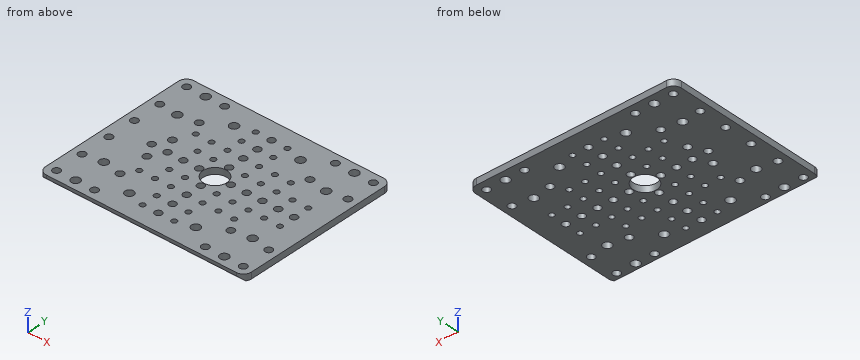
```python
from build123d import *

# Parameters (mm, degrees)
SKETCH_W        = 130
SKETCH_H        = 104
PAD_DEPTH       = 4
SKETCH001_R     = 2.35
SKETCH001_R_2   = 2.75
POCKET_DEPTH    = 4.001
SKETCH002_R     = 1.7
SKETCH002_R_2   = 2.25
SKETCH002_R_3   = 7.5
POCKET001_DEPTH = 5
CHAMFER_SIZE    = 2
FILLET_R        = 5


with BuildPart() as part:
    # Sketch → Pad (new body)
    with BuildSketch(Plane.XY):
        Rectangle(SKETCH_W, SKETCH_H)
    extrude(amount=PAD_DEPTH)

    # Sketch001 → Pocket (cut, through all)
    with BuildSketch(Plane.XY.offset(4)):
        with Locations((-35, 46)):
            Circle(SKETCH001_R)
        with Locations((-59, 27)):
            Circle(SKETCH001_R)
        with Locations((-59, 46)):
            Circle(SKETCH001_R)
        with Locations((35, 46)):
            Circle(SKETCH001_R)
        with Locations((59, 28)):
            Circle(SKETCH001_R)
        with Locations((59, 46)):
            Circle(SKETCH001_R)
        with Locations((59, -28)):
            Circle(SKETCH001_R)
        with Locations((59, -46)):
            Circle(SKETCH001_R)
        with Locations((35, -46)):
            Circle(SKETCH001_R)
        with Locations((-59, -28)):
            Circle(SKETCH001_R)
        with Locations((-35, -46)):
            Circle(SKETCH001_R)
        with Locations((-59, -46)):
            Circle(SKETCH001_R)
        with Locations((-47, 46)):
            Circle(SKETCH001_R_2)
        with Locations((-47, 26)):
            Circle(SKETCH001_R_2)
        with Locations((47, 46)):
            Circle(SKETCH001_R_2)
        with Locations((47, 26)):
            Circle(SKETCH001_R_2)
        with Locations((-21, -37)):
            Circle(SKETCH001_R_2)
        with Locations((21, -37)):
            Circle(SKETCH001_R_2)
        with Locations((-21, 37)):
            Circle(SKETCH001_R_2)
        with Locations((21, 37)):
            Circle(SKETCH001_R_2)
        with Locations((47, -46)):
            Circle(SKETCH001_R_2)
        with Locations((47, -26)):
            Circle(SKETCH001_R_2)
        with Locations((-47, -26)):
            Circle(SKETCH001_R_2)
        with Locations((-47, -46)):
            Circle(SKETCH001_R_2)
        with Locations((-35, 28)):
            Circle(SKETCH001_R)
        with Locations((35, 28)):
            Circle(SKETCH001_R)
        with Locations((35, -28)):
            Circle(SKETCH001_R)
        with Locations((-35, -28)):
            Circle(SKETCH001_R)
        with Locations((-59, 9)):
            Circle(SKETCH001_R)
        with Locations((-59, -9)):
            Circle(SKETCH001_R)
        with Locations((-35, 9)):
            Circle(SKETCH001_R)
        with Locations((-35, -9)):
            Circle(SKETCH001_R)
    extrude(amount=-POCKET_DEPTH, mode=Mode.SUBTRACT)

    # Sketch002 → Pocket001 (cut)
    with BuildSketch(Plane.XY.offset(4)):
        with Locations((-10, 10)):
            Circle(SKETCH002_R)
        with Locations((-20, 10)):
            Circle(SKETCH002_R)
        with Locations((-10, 0)):
            Circle(SKETCH002_R_2)
        with Locations((-20, 0)):
            Circle(SKETCH002_R_2)
        with Locations((-10, -10)):
            Circle(SKETCH002_R)
        with Locations((-20, -10)):
            Circle(SKETCH002_R)
        with Locations((-30, 0)):
            Circle(SKETCH002_R_2)
        with Locations((-40, 0)):
            Circle(SKETCH002_R_2)
        with Locations((10, 10)):
            Circle(SKETCH002_R)
        with Locations((10, -10)):
            Circle(SKETCH002_R)
        with Locations((20, -10)):
            Circle(SKETCH002_R)
        with Locations((20, 10)):
            Circle(SKETCH002_R)
        with Locations((30, 10)):
            Circle(SKETCH002_R)
        with Locations((40, 10)):
            Circle(SKETCH002_R)
        with Locations((30, -10)):
            Circle(SKETCH002_R)
        with Locations((40, -10)):
            Circle(SKETCH002_R)
        with Locations((-10, 20)):
            Circle(SKETCH002_R)
        with Locations((-20, 20)):
            Circle(SKETCH002_R)
        with Locations((10, 20)):
            Circle(SKETCH002_R)
        with Locations((20, 20)):
            Circle(SKETCH002_R)
        with Locations((20, -20)):
            Circle(SKETCH002_R)
        with Locations((10, -20)):
            Circle(SKETCH002_R)
        with Locations((-10, -20)):
            Circle(SKETCH002_R)
        with Locations((-20, -20)):
            Circle(SKETCH002_R)
        with Locations((-10, 30)):
            Circle(SKETCH002_R)
        with Locations((-10, 40)):
            Circle(SKETCH002_R)
        with Locations((10, 40)):
            Circle(SKETCH002_R)
        with Locations((10, 30)):
            Circle(SKETCH002_R)
        with Locations((10, -30)):
            Circle(SKETCH002_R)
        with Locations((-10, -30)):
            Circle(SKETCH002_R)
        with Locations((-10, -40)):
            Circle(SKETCH002_R)
        with Locations((10, -40)):
            Circle(SKETCH002_R)
        with Locations((0, 40)):
            Circle(SKETCH002_R_2)
        with Locations((0, 30)):
            Circle(SKETCH002_R_2)
        with Locations((0, 20)):
            Circle(SKETCH002_R_2)
        with Locations((0, 10)):
            Circle(SKETCH002_R_2)
        with Locations((0, -10)):
            Circle(SKETCH002_R_2)
        with Locations((0, -20)):
            Circle(SKETCH002_R_2)
        with Locations((0, -30)):
            Circle(SKETCH002_R_2)
        with Locations((0, -40)):
            Circle(SKETCH002_R_2)
        with Locations((10, 0)):
            Circle(SKETCH002_R_2)
        with Locations((20, 0)):
            Circle(SKETCH002_R_2)
        with Locations((30, 0)):
            Circle(SKETCH002_R_2)
        with Locations((40, 0)):
            Circle(SKETCH002_R_2)
        with Locations((50, 0)):
            Circle(SKETCH002_R_2)
        with Locations((50, 10)):
            Circle(SKETCH002_R)
        with Locations((50, -10)):
            Circle(SKETCH002_R)
        with Locations((-30, 20)):
            Circle(SKETCH002_R)
        with Locations((-30, -20)):
            Circle(SKETCH002_R)
        with Locations((30, 20)):
            Circle(SKETCH002_R)
        with Locations((30, -20)):
            Circle(SKETCH002_R)
        Circle(SKETCH002_R_3)
    extrude(amount=-POCKET001_DEPTH, mode=Mode.SUBTRACT)

    # Chamfer
    chamfer_edges = [part.edges().sort_by_distance(p)[0] for p in [
        (0, -52, 0),
    ]]
    chamfer(chamfer_edges, length=CHAMFER_SIZE)

    # Fillet
    fillet_edges = [part.edges().sort_by_distance(p)[0] for p in [
        (-65, 52, 2),
        (-65, -52, 3),
        (65, -52, 3),
        (65, 52, 2),
    ]]
    fillet(fillet_edges, radius=FILLET_R)


solid = part.part
```
Geometry check sheet. Reference: the model listing, model coordinates, mm. Coordinates: 2 decimals unless noted, no trailing zeros. Write each loop counter-clockwise with the first axis right and the second up, starting at its lowest first coordinate (ties: lowest second). Pieces come first, ordered by that corner, then holes. Notation, with made-up numbers: (86.5, 1.5) -> (115.5, 1.5) arc R27 ccw to (115.5, 24.5) -> close; hole circle Ø10 at (25.25, 74). An arc over 180 degrees is marked (long way). Use CSV: the item, a comma, the result in double quotes. Start each with the question number.
Item 1: Cross-section at A-A, the plane x = -30. Record the cut outline in (y, z), plus the area to 3 significant figures.
Item 2: Thickness scan on line 1 (X direction, y = 39, z = 0.8); line 2 (Y direction, x = 33.5, z = 2); line 3 (Y direction, x = 38.5, z = 0.8). Record the ranges inside material, lowest first.
Item 3: Cross-section at B-B, the plane y = -20. State how many separate pieces and enclosed holes the cut face has, plus the area to 3 significant figures.
Answers:
1,outline,"(-52, 2) -> (-50, 0) -> (-21.7, 0) -> (-21.7, 4) -> (-52, 4) -> close; (-18.3, 0) -> (-2.25, 0) -> (-2.25, 4) -> (-18.3, 4) -> close; (2.25, 0) -> (18.3, 0) -> (18.3, 4) -> (2.25, 4) -> close; (21.7, 0) -> (52, 0) -> (52, 4) -> (21.7, 4) -> close"
1,area,"369 mm^2"
2,line 1,"-65 to -22.89, -19.11 to -11.37, -8.63 to -2.02, 2.02 to 8.63, 11.37 to 19.11, 22.89 to 65"
2,line 2,"-52 to -47.81, -44.19 to -29.81, -26.19 to 26.19, 29.81 to 44.19, 47.81 to 52"
2,line 3,"-50.8 to -10.8, -9.2 to -1.68, 1.68 to 9.2, 10.8 to 52"
3,separate pieces,"8"
3,enclosed holes,"0"
3,area,"420 mm^2"
